Verification items for this drawing (mm, ordinates from the low corner). A direction names the side the tool comes from. Coordinates: 2 decimals unless noted, no trailing zeros. Write each loop counter-clockwise with the first axis right and the second up, starting at its lowest first coordinate (ties: lowest second). Pieces come first, ordered by that corner, then holes. Notation, with made-up numbers: M 20,-23.75 L 30,-23.75 A29 ccw 30,-2.75 Z; hole C 40.5,12.5 d8. An arc over 180 degrees is marked long. Put each result on its own line as item: value. Start each with the question number.
1) Gauge pin test, flat ends, axial feed: pin 1 (3 mm diameter, centred on x = 51, z = 5, fed in from +Y); pin 2 (3 mm diameter, centred on x = 38.5, y = 12, fed in from -Z); pin 3 (3.5 mm diameter, centred on x = 52, y = 4, fed in from -Z); pin 4 (2 mm diameter, centred on x = 32.5, y = 11, fed in from -Z). Record the tip position at first contact, or that the pin passes through.
2) Cross-section at B-B on y = 4. Record the cut outline in (x, z), plus the area to 3 significant figures.
3) Mould release check, pull along Y, two halves, no side actions. Record for the marked faces 1, 2 and 3: released by +Y, released by -Y, zero draft, split by the parting line, or undercut.
4) Cross-section at C-C on z = 4.5. Record the cut outline in (x, y).
5) Scan lines: line 1 along Y through (x, z) = (4, 3.5); line 2 along Y through (x, z) = (38.5, 7.5); line 3 along X through (y, z) = (5.75, 8.25). Record each from-to range of solid material in increasing order.
6) Cross-section at D-D on z = 11.5. Record the cut outline in (x, y).
7) Cross-section at A-A on x = 52. Record the cut outline in (y, z), plus the area to 4 significant figures.
8) Set-up check for the marked faces 4, 5, 6, 7 and 8: record each of +Z, -Z, +X, -X, +Y, -Y from which the full face is reachable in a straight line by a thin tool's end or side.
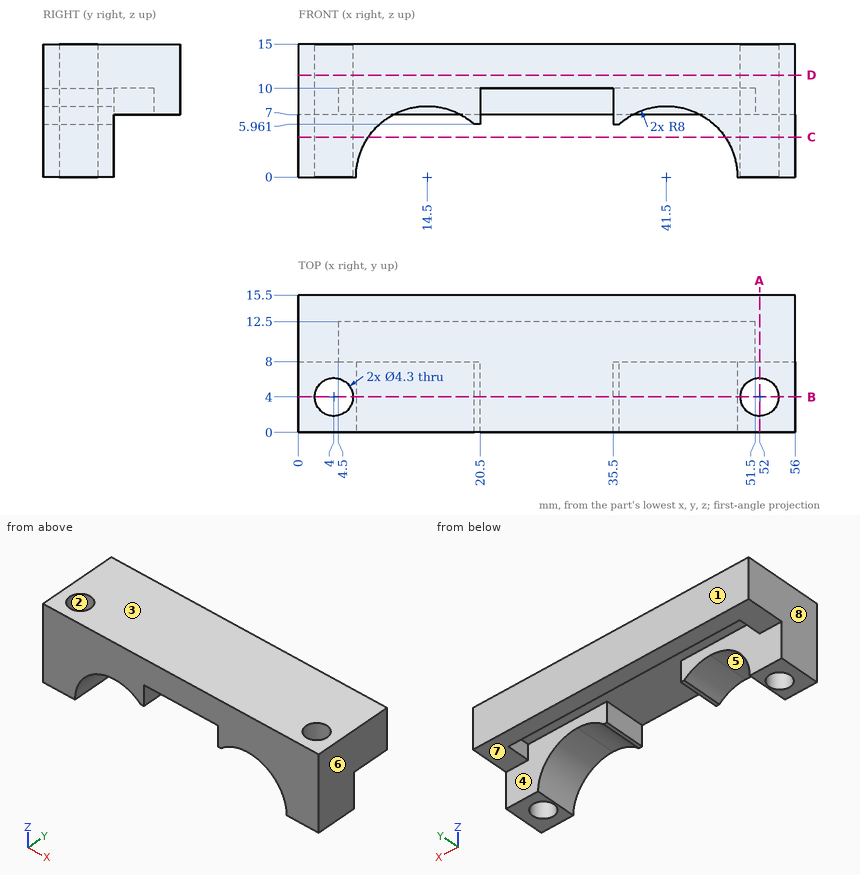
Answer key:
1. pin 1: stops at y = 8
1. pin 2: stops at z = 7
1. pin 3: passes through
1. pin 4: stops at z = 10
2. outline: M 0,0 L 1.85,0 L 1.85,15 L 0,15 Z; M 6.15,0 L 6.5,0 A8 cw 14.5,8 A8 cw 19.84,5.96 L 20.5,5.96 L 20.5,10 L 35.5,10 L 35.5,5.96 L 36.16,5.96 A8 cw 41.5,8 A8 cw 49.5,0 L 49.85,0 L 49.85,15 L 6.15,15 Z; M 54.15,0 L 56,0 L 56,15 L 54.15,15 Z
2. area: 374 mm²
3. face 1: released by +Y
3. face 2: undercut
3. face 3: zero draft
4. outline: M 0,0 L 7.89,0 L 7.89,8 L 0,8 Z; M 48.11,0 L 56,0 L 56,8 L 48.11,8 Z; hole C 4,4 d4.3; hole C 52,4 d4.3
5. line 1: y = 0 to 1.85, 6.15 to 8
5. line 2: y = 0 to 8, 12.5 to 15.5
5. line 3: x = 0 to 2.75, 5.25 to 20.5, 35.5 to 50.75, 53.25 to 56
6. outline: M 0,0 L 56,0 L 56,15.5 L 0,15.5 Z; hole C 4,4 d4.3; hole C 52,4 d4.3
7. outline: M 0,0 L 1.85,0 L 1.85,15 L 0,15 Z; M 6.15,0 L 8,0 L 8,7 L 15.5,7 L 15.5,15 L 6.15,15 Z
7. area: 115.5 mm²
8. face 4: -Z
8. face 5: -Z, -Y
8. face 6: +Z, -Z, +X, +Y, -Y
8. face 7: -Z, +X, -X, +Y
8. face 8: +Z, -Z, -X, +Y, -Y
